The model under review builds one solid part; all positions refer to its coordinate system, in mm. A direction names the side the tool comes from. Coordinates: 2 decimals unless noted, no trailing zeros. Write each loop counter-clockwise with the first axis right and the second up, starting at its lowest first coordinate (ties: lowest second). Pieces come first, ordered by that corner, then holes.
1) Mouldability with a two-part tool opening along Y and no side actions: class faces 5 (the cylindrical face through (-95.059, -12.325, -6.774)), 6 (the cylindrical face through (-9.941, 34.65, -6.774)), 7 (the flat face through (-51, 10, -10)), 8 (the flat face through (-90, -35, -10)) as released by +Y, released by -Y, zero draft, split by the parting line, or undercut.
2) Add section B-B, the plane x = -63.5. State the section outline as (y, z) points, then the cut area to 3 significant figures.
3) Add section C-C, the plane z = -10. State the section outline as (x, y) points, then the cut area to 3 significant figures.
4) For P1, Ø5, axis at x = -74, y = 4, coming from the -Z side; P2, Ø12, axis at x = -69.5, z = 27, coming from the +Y side; P3, Ø8, axis at y = 6, z = -14, coming from the -X side, all flat-tipped, find the tip position at first contact; note any pin that passes through.
5) Add section A-A, the plane x = -15. State the section outline as (y, z) points.
6) Machinability: for faces 1 (the flat face through (-100, 5, -10)), 2 (the flat face through (-102, -30, -38)), 3 (the flat face through (-51, 5, 0)), 4 (the flat face through (-51, 5, -20)), which of the approach directions +Z, -Z, +X, -X, +Y, -Y give a long, thin tool a straight path to every point of the face, cutting with its end or side? Answer none if there is none.
7) Add section D-D, the plane y = -4.5. State the section outline as (x, z) points, then the cut area to 3 significant figures.
8) For line 1 (Y direction, x = -134, z = -41.5); line 2 (Y direction, x = -22, z = -18.5); line 3 (Z direction, x = -89.5, y = 0.5), list the stretches that pass through material, from the lowest coordinate up.
from build123d import *

# Parameters (mm, degrees)
SKETCH_1_W      = 100
SKETCH_1_H      = 20
EXTRUDE_1_DEPTH = 10
SKETCH_4_R      = 6
EXTRUDE_2_DEPTH = 50
SKETCH_6_R      = 6
EXTRUDE_3_DEPTH = 30
SKETCH_7_R      = 30
EXTRUDE_4_DEPTH = 5
SKETCH_8_R      = 60
EXTRUDE_5_DEPTH = 5


with BuildPart() as part:
    # ｽｹｯﾁ1 → ﾎﾞｽ - 押し出し1 (new body)
    with BuildSketch(Plane(origin=(0, 0, 0), x_dir=(1, 0, 0), z_dir=(0, 1, 0))):
        with Locations((-50, 10)):
            Rectangle(SKETCH_1_W, SKETCH_1_H)
    extrude(amount=EXTRUDE_1_DEPTH)

    # ｽｹｯﾁ4 → ﾎﾞｽ - 押し出し2 (add)
    with BuildSketch(Plane(origin=(0, 10, 0), x_dir=(1, 0, 0), z_dir=(0, 1, 0))):
        with Locations(Location((-15, 10, 0), (0, 0, 270))):
            Circle(SKETCH_4_R)
    extrude(amount=EXTRUDE_2_DEPTH)

    # ｽｹｯﾁ6 → ﾎﾞｽ - 押し出し3 (add)
    with BuildSketch(Plane.XZ):
        with Locations(Location((-90, -10, 0), (0, 0, 90))):
            Circle(SKETCH_6_R)
    extrude(amount=EXTRUDE_3_DEPTH)

    # ｽｹｯﾁ7 → ﾎﾞｽ - 押し出し4 (add)
    with BuildSketch(Plane.XZ.offset(30)):
        with Locations(Location((-90, -10, 0), (0, 0, 270))):
            Circle(SKETCH_7_R)
    extrude(amount=EXTRUDE_4_DEPTH)

    # ｽｹｯﾁ8 → ﾎﾞｽ - 押し出し5 (add)
    with BuildSketch(Plane(origin=(0, -30, 0), x_dir=(1, 0, 0), z_dir=(0, 1, 0))):
        with Locations(Location((-90, 10, 0), (0, 0, 270))):
            Circle(SKETCH_8_R)
    extrude(amount=EXTRUDE_5_DEPTH)


solid = part.part
Geometry results:
1. face 5: undercut
1. face 6: zero draft
1. face 7: released by +Y
1. face 8: released by -Y
2. outline: (-35, -24.06) - (-30, -24.06) - (-30, -63.83) - (-25, -63.83) - (-25, 43.83) - (-30, 43.83) - (-30, 4.06) - (-35, 4.06) - close; (0, -20) - (10, -20) - (10, 0) - (0, 0) - close
2. area: 879 mm2
3. outline: (-150, -30) - (-120, -30) - (-120, -35) - (-60, -35) - (-60, -30) - (-30, -30) - (-30, -25) - (-84, -25) - (-84, 0) - (0, 0) - (0, 10) - (-9, 10) - (-9, 60) - (-21, 60) - (-21, 10) - (-100, 10) - (-100, 0) - (-96, 0) - (-96, -25) - (-150, -25) - close
3. area: 2,800 mm2
4. P1: stops at z = -20
4. P2: stops at y = -25
4. P3: stops at x = -100
5. outline: (0, -20) - (10, -20) - (10, -16) - (60, -16) - (60, -4) - (10, -4) - (10, 0) - (0, 0) - close
6. face 1: +Z, -Z, -X, +Y
6. face 2: -Y
6. face 3: +Z, +X, -X, +Y
6. face 4: -Z, +X, -X, +Y
7. outline: circle Ø12 at (-90, -10)
7. area: 113 mm2
8. line 1: y = -30 to -25
8. line 2: y = 0 to 10
8. line 3: z = -20 to 0
